```python
from build123d import *

# Parameters (mm, degrees)
SKETCH3_R          = 12.26998913
CUT_EXTRUDE1_DEPTH = 10
FILLET1_R          = 10
SKETCH4_R          = 2.26998913
CUT_EXTRUDE2_DEPTH = 10


with BuildPart() as part:
    # Sketch1 → Revolve1 (revolve)
    with BuildSketch(Plane.XY, mode=Mode.PRIVATE) as revolve1_sk:
        Polygon((558.630730273, 31.133640952), (561.480624089, 42.622275397), (570.080624089, 42.622275397), (570.080624089, 6.108010882), (552.040350824, 6.108010882), (556.849546639, 31.133640952), align=None)
    revolve(revolve1_sk.sketch.rotate(Axis((570.080624089, 6.108010882, 0), (0, 1, 0)), 270), axis=Axis((570.080624089, 6.108010882, 0), (0, 1, 0)))

    # Sketch3 → Cut-Extrude1 (cut)
    with BuildSketch(Plane(origin=(0, 6.108010882, 0), x_dir=(-1, 0, 0), z_dir=(0, -1, 0))):
        with Locations(Location((-570.080624089, 0, 0), (0, 0, 90))):
            Circle(SKETCH3_R)
    extrude(amount=-CUT_EXTRUDE1_DEPTH, mode=Mode.SUBTRACT)

    # Fillet1
    fillet1_edges = [part.edges().sort_by_distance(p)[0] for p in [
        (570.080624089, 16.108010882, 12.26998913),
    ]]
    fillet(fillet1_edges, radius=FILLET1_R - 0.0001)  # a hair under: the kernel refuses the full size

    # Sketch4 → Cut-Extrude2 (cut)
    with BuildSketch(Plane(origin=(0, 16.108010882, 0), x_dir=(-1, 0, 0), z_dir=(0, -1, 0))):
        with Locations(Location((-570.080624089, 0, 0), (0, 0, 90))):
            Circle(SKETCH4_R)
    extrude(amount=-CUT_EXTRUDE2_DEPTH, mode=Mode.SUBTRACT)


solid = part.part
```
CAD build for the part. Positions are in the model's coordinates, mm. Give positions to 0.01 mm unless a question says otherwise; leave off trailing zeros. Loops run counter-clockwise (first coordinate to the right, second up) from the corner with the lowest first, then second, coordinate; pieces in that order, holes last. Notation, with made-up numbers: (46.5, -34.5) -> (63.5, -34.5) arc R12 cw to (63.5, -14.5) -> close; hole circle Ø2 at (33.25, 5). An arc over 180 degrees is marked (long way). Use a Markdown table: item, result.
1. Wall check: L1, parallel to Y at x = 582.5, z = 0.5; L2, parallel to X at y = 22.75, z = 0; L3, parallel to Y at x = 572.5, z = 1. Give the ranges that are in metal, low to high. Write a range as [from, to].
Check result:
| item | result |
|---|---|
| L1 | y = [6.11, 31.13] |
| L2 | x = [555.24, 567.81], [572.35, 584.92] |
| L3 | y = [16.1, 42.62] |
2. Mould opens along Z. For faces 1 (the conical face through (579.23, 39.51, 2.03)), 2 (the flat face through (560, 31.134, 6)), 3 (the flat face through (570, 26.108, 0)), 4 (the cylindrical face through (571.995, 21.038, -1.22)) say: pulls with the +Z half, pulls with the -Z half, needs draft (parallel to the pull), parting line crosses it, or undercut.
Check result:
| item | result |
|---|---|
| face 1 | parting line crosses it |
| face 2 | needs draft |
| face 3 | undercut |
| face 4 | undercut |
3. Flat gauge pins, fed straight in: pin 1 (1.5 mm diameter, centred on y = 17.5, z = -9, fed in from +X); pin 2 (3 mm diameter, centred on y = 31.5, z = -2, fed in from -X); pin 3 (4 mm diameter, centred on x = 578.5, y = 20, fed in from -Z). Where does each tip first touch, or does it go through?
Check result:
| item | result |
|---|---|
| pin 1 | stops at x = 583.65 |
| pin 2 | stops at x = 556.73 |
| pin 3 | stops at z = -14.06 |
4. Slice it at B-B (y = 37). List the corners of the cut face in (x, z), plus the area to 3 significant figures.
Check result:
| item | result |
|---|---|
| outline | circle Ø19.99 at (570.08, 0) |
| area | 314 mm^2 |
5. Slice it at A-A (y = 25). List the corners of the cut face in (x, z).
Check result:
| item | result |
|---|---|
| outline | circle Ø28.82 at (570.08, 0); hole circle Ø4.54 at (570.08, 0) |
